Can you work these out from the model? Positions are in its coordinate system, mm. Face numbers are marked on the shaded views. Give positions to 0.01 mm unless a question says otherwise; leave off trailing zeros. Order: outer loops, then holes, each group sorted by start corner. A loop starts at its lowest first (then second) coordinate and runs counter-clockwise, first axis right, second up. Notation, with made-up numbers: (86.25, 78.25) - (119.25, 78.25) arc R6 ccw to (119.25, 88.25) - close; hole circle Ø8 at (64.25, 56). An arc over 180 degrees is marked (long way). Return JSON: item names as keys, results as strings.
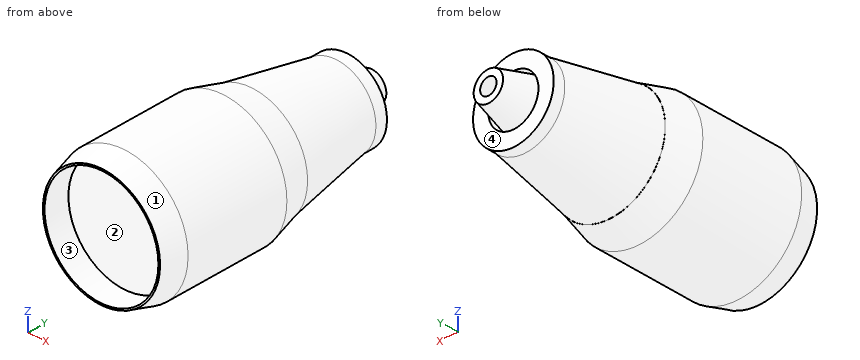
```python
from build123d import *

# Parameters (mm, degrees)
F0_R          = 26.3014880092
F0_R_2        = 23.0827140561
F1_DEPTH      = 39.878
F1_DEPTH_BACK = 25.4
F2_DEPTH      = 14.986
F3_DEPTH      = 76.708
F5_SIZE2      = 3.4029547439
F5_SIZE       = 12.7
F6_SIZE2      = 9.4794090512
F6_SIZE       = 2.54
F7_R          = 13.5748533888
F8_DEPTH      = 15.748
F10_T         = -2.54
F11_DEPTH     = 4.826


# Not quite as in the source:
# - a fillet or chamfer that OpenCascade refuses, or shapes differently, is made with other operations: its cross-section is extruded or revolved along the edge and cut away or added


with BuildPart() as f1:
    # F0 (on Front) → F1 (new body, two sides)
    with BuildSketch(Plane.XZ) as f1_sk:
        Circle(F0_R)
        Circle(F0_R_2, mode=Mode.SUBTRACT)
    extrude(amount=-F1_DEPTH)
    extrude(f1_sk.sketch, amount=F1_DEPTH_BACK)

    # F0 (on Front) → F2 (join)
    with BuildSketch(Plane.XZ):
        Circle(F0_R_2)
    extrude(amount=F2_DEPTH)

    # F0 (on Front) → F3 (join)
    with BuildSketch(Plane.XZ):
        Circle(F0_R_2)
    extrude(amount=-F3_DEPTH)

    # F4: chamfer of 38.1 x 6.718057965 on 1 edges, made by hand


with BuildPart() as f4_tool2:
    # F4_s3 → F4_t4 (revolve)
    with BuildSketch(Plane.XY):
        Polygon((23.0827140561, 38.608), (16.3646560911, 76.708), (23.0827140561, 76.708), align=None)
    revolve(axis=Axis((0, 76.708, 0), (0, -1, 0)))

    split(bisect_by=Plane.XZ.offset(-39.878), keep=Keep.BOTTOM)


with BuildPart() as f1_1:
    add(f1.part)

    # F4_t1: cut F4_tool2
    add(f4_tool2.part, mode=Mode.SUBTRACT)

    # F5
    f5_edges = [f1_1.edges().sort_by_distance(p)[0] for p in [
        (-26.301488, 39.878, 0),
    ]]
    f5_side = f1_1.faces().sort_by_distance((-26.301488, 7.239, 0))[0]
    chamfer(f5_edges, length=F5_SIZE, length2=F5_SIZE2, reference=f5_side)

    # F6
    f6_edges = [f1_1.edges().sort_by_distance(p)[0] for p in [
        (-26.301488, -25.4, 0),
    ]]
    f6_side = f1_1.faces().sort_by_distance((-25.55757, -25.4, 0))[0]
    chamfer(f6_edges, length=F6_SIZE, length2=F6_SIZE2, reference=f6_side)

    # F7 (on face) → F8 (join)
    with BuildSketch(Plane(origin=(0, 76.708, 0), x_dir=(-1, 0, 0), z_dir=(0, 1, 0))):
        Circle(F7_R)
    extrude(amount=F8_DEPTH)

    # F9: chamfer of 7.62 x 28.4382271537 on 1 edges, made by hand


with BuildPart() as f9_tool2:
    # F9_s3 → F9_t4 (revolve)
    with BuildSketch(Plane.XY):
        Polygon((-13.5748533888, 64.0177728463), (-5.9548533888, 92.456), (-13.5748533888, 92.456), align=None)
    revolve(axis=Axis((0, 92.456, 0), (0, 1, 0)))

    split(bisect_by=Plane.XZ.offset(-76.708), keep=Keep.BOTTOM)


with BuildPart() as f1_2:
    add(f1_1.part)

    # F9_t1: cut F9_tool2
    add(f9_tool2.part, mode=Mode.SUBTRACT)

    # F10
    f10_openings = [f1_2.faces().sort_by_distance(p)[0] for p in [
        (0, 92.456, 0),
    ]]
    offset(amount=F10_T, openings=f10_openings, kind=Kind.INTERSECTION)

    # F11 (add): a face of the model
    f11_faces = [f1_2.faces().sort_by_distance(p)[0] for p in [
        (-15.9017937193, 76.708, 0),
    ]]
    extrude(f11_faces, amount=F11_DEPTH)


solid = f1_2.part
```
1. Suppose I cut it at C-C (y = 42.5). List the corners of the cut face in (x, z) for me.
Checks:
{"outline": "circle Ø44.79 at (0, 0); hole circle Ø39.63 at (0, 0)"}
2. For pin 1 Ø1 at (y, z) = (-5, 11.5) entering from -X; pin 2 Ø14 at (x, z) = (-5, 0) entering from -Y; pin 3 Ø3 at (x, z) = (13, 7) entering from +Y, each with a flat end and sliding along its axis, tell me the tip position at first contact or that it passes through.
Checks:
{"pin 1": "x = -23.89", "pin 2": "y = -14.99", "pin 3": "y = 81.53"}
3. Thinking about a two-plate mould opening in X: for the marked faces 1, 2, 3 and 4, which applies, +X half, -X half, draft (parallel to the pull), parting line (faces both ways), or undercut?
Checks:
{"face 1": "parting line", "face 2": "undercut", "face 3": "undercut", "face 4": "draft"}
4. Suppose I cut it at B-B (y = 61). List the corners of the cut face in (x, z) for me.
Checks:
{"outline": "circle Ø38.27 at (0, 0); hole circle Ø33.11 at (0, 0)"}
5. If I drill on L1, parallel to Z at x = 0, y = 78; L2, parallel to Z at x = 0, y = 79.45; L3, parallel to Y at x = 0, z = 11, over which ranges is the centre line in solid material (lowest first)? Write a range as [from, to].
Checks:
{"L1": "[-16.36, -10.17], [-9.83, -7.2], [7.2, 9.83], [10.17, 16.36]", "L2": "[-16.36, -10.17], [-9.44, -6.81], [6.81, 9.44], [10.17, 16.36]", "L3": "[-14.99, -12.45], [74.17, 81.53]"}
6. Suppose I cut it at A-A (y = 80). List the corners of the cut face in (x, z) for me, plus the area to 3 significant figures.
Checks:
{"outline": "circle Ø32.73 at (0, 0); circle Ø18.58 at (0, 0); hole circle Ø20.35 at (0, 0); hole circle Ø13.33 at (0, 0)", "area": "648 mm^2"}
